The listing builds one solid part. Answer for the finished solid, in the listing's coordinates (mm). A direction names the side the tool comes from. Coordinates: 2 decimals unless noted, no trailing zeros. Loops run counter-clockwise (first coordinate to the right, second up) from the corner with the lowest first, then second, coordinate; pieces in that order, holes last. Notation, with made-up numbers: (44.25, 8) -> (77.25, 8) arc R13 cw to (77.25, 27) -> close; hole circle Ø5 at (39.25, 1). An arc over 180 degrees is marked (long way). Answer in a Markdown table with one row per item.
```python
from build123d import *

# Parameters (mm, degrees)
SKETCH1_R           = 10.5
SKETCH1_R_2         = 1.5
BOSS_EXTRUDE1_DEPTH = 2
SKETCH2_R           = 4.4
SKETCH2_R_2         = 3
BOSS_EXTRUDE2_DEPTH = 3.7
SKETCH3_R           = 0.75
CUT_EXTRUDE1_DEPTH  = 10


with BuildPart() as part:
    # Sketch1 → Boss-Extrude1 (new body)
    with BuildSketch(Plane(origin=(0, 0, 0), x_dir=(1, 0, 0), z_dir=(0, 1, 0))):
        with Locations(Location((0, 0, 0), (0, 0, 270))):
            Circle(SKETCH1_R)
        with Locations(Location((0, 0, 0), (0, 0, 270))):
            Circle(SKETCH1_R_2, mode=Mode.SUBTRACT)
    extrude(amount=-BOSS_EXTRUDE1_DEPTH)

    # Sketch2 → Boss-Extrude2 (add)
    with BuildSketch(Plane.XZ.offset(2)):
        with Locations(Location((0, 0, 0), (0, 0, 90))):
            Circle(SKETCH2_R)
        with Locations(Location((0, 0, 0), (0, 0, 270))):
            Circle(SKETCH2_R_2, mode=Mode.SUBTRACT)
    extrude(amount=BOSS_EXTRUDE2_DEPTH)

    # Sketch3 → Cut-Extrude1 (cut)
    with BuildSketch(Plane(origin=(0, 0, 0), x_dir=(1, 0, 0), z_dir=(0, 1, 0))):
        with Locations(Location((0, 7.25, 0), (0, 0, 270))):
            Circle(SKETCH3_R)
        with Locations(Location((3.5, 7.25, 0), (0, 0, 270))):
            Circle(SKETCH3_R)
        with Locations(Location((-3.5, 7.25, 0), (0, 0, 270))):
            Circle(SKETCH3_R)
        with Locations(Location((-7.25, 3.5, 0), (0, 0, 270))):
            Circle(SKETCH3_R)
        with Locations(Location((-7.25, -3.5, 0), (0, 0, 270))):
            Circle(SKETCH3_R)
        with Locations(Location((-7.25, 0, 0), (0, 0, 270))):
            Circle(SKETCH3_R)
        with Locations(Location((7.25, -3.5, 0), (0, 0, 270))):
            Circle(SKETCH3_R)
        with Locations(Location((7.25, 3.5, 0), (0, 0, 270))):
            Circle(SKETCH3_R)
        with Locations(Location((7.25, 0, 0), (0, 0, 270))):
            Circle(SKETCH3_R)
        with Locations(Location((0, -7.25, 0), (0, 0, 270))):
            Circle(SKETCH3_R)
        with Locations(Location((-3.5, -7.25, 0), (0, 0, 270))):
            Circle(SKETCH3_R)
        with Locations(Location((3.5, -7.25, 0), (0, 0, 270))):
            Circle(SKETCH3_R)
    extrude(amount=-CUT_EXTRUDE1_DEPTH, mode=Mode.SUBTRACT)


solid = part.part
```
Item 1: A tool of negligible diameter and unlimited length cuts with its end or side. For faces 4 (the face through (-1.3, -2, 1.3)), 5 (the face through (3.2, -1, 10)), from which of +Z, -Z, +X, -X, +Y, -Y can it reach the whole face along a straight path? Write none if from no direction.
Findings below:
| item | result |
|---|---|
| face 4 | -Y |
| face 5 | +Y, -Y |
Item 2: Find the intervals of material crossed by probe 1 along X at (y, z) = (-0.35, 4); probe 2 along Y at (x, z) = (-7.5, 2); probe 3 along X at (y, z) = (-1.5, 7.25), in increasing order.
Findings below:
| item | result |
|---|---|
| probe 1 | x = -9.71 to -7.81, -6.69 to 6.69, 7.81 to 9.71 |
| probe 2 | y = -2 to 0 |
| probe 3 | x = -7.6 to -4.25, -2.75 to -0.75, 0.75 to 2.75, 4.25 to 7.6 |
Item 3: A cutting plane is placed at A-A, the plane x = 0. Determine the outline of the cut face in (y, z), plus the area to 3 significant figures.
Findings below:
| item | result |
|---|---|
| outline | (-5.7, -4.4) -> (-2, -4.4) -> (-2, -6.5) -> (0, -6.5) -> (0, -1.5) -> (-2, -1.5) -> (-2, -3) -> (-5.7, -3) -> close; (-5.7, 3) -> (-2, 3) -> (-2, 1.5) -> (0, 1.5) -> (0, 6.5) -> (-2, 6.5) -> (-2, 4.4) -> (-5.7, 4.4) -> close; (-2, -10.5) -> (0, -10.5) -> (0, -8) -> (-2, -8) -> close; (-2, 8) -> (0, 8) -> (0, 10.5) -> (-2, 10.5) -> close |
| area | 40.4 mm2 |
Item 4: A cutting plane is placed at B-B, the plane z = 0. Determine the outline of the cut face in (x, y), plus the area to 3 significant figures.
Findings below:
| item | result |
|---|---|
| outline | (-10.5, -2) -> (-8, -2) -> (-8, 0) -> (-10.5, 0) -> close; (-6.5, -2) -> (-4.4, -2) -> (-4.4, -5.7) -> (-3, -5.7) -> (-3, -2) -> (-1.5, -2) -> (-1.5, 0) -> (-6.5, 0) -> close; (1.5, -2) -> (3, -2) -> (3, -5.7) -> (4.4, -5.7) -> (4.4, -2) -> (6.5, -2) -> (6.5, 0) -> (1.5, 0) -> close; (8, -2) -> (10.5, -2) -> (10.5, 0) -> (8, 0) -> close |
| area | 40.4 mm2 |
Item 5: A cutting plane is placed at D-D, the plane x = -3.25. Determine the outline of the cut face in (y, z), plus the area to 3 significant figures.
Findings below:
| item | result |
|---|---|
| outline | (-5.7, -2.97) -> (-2, -2.97) -> (-2, -6.54) -> (0, -6.54) -> (0, 6.54) -> (-2, 6.54) -> (-2, 2.97) -> (-5.7, 2.97) -> close; (-2, -9.98) -> (0, -9.98) -> (0, -7.96) -> (-2, -7.96) -> close; (-2, 7.96) -> (0, 7.96) -> (0, 9.98) -> (-2, 9.98) -> close |
| area | 56.2 mm2 |
Item 6: Determine the mould class of faces 1 (the face through (0, 0, 2)), 2 (the face through (-4.363, -3.824, -0.573)), 3 (the face through (0.9, -3.82, -2.86)) for opening direction X: +X half, -X half, draft (parallel to the pull), parting line (faces both ways), or undercut.
Findings below:
| item | result |
|---|---|
| face 1 | draft |
| face 2 | parting line |
| face 3 | undercut |
Item 7: Flat-ended cylindrical pins translate along their axes: pin 1 Ø3 at (y, z) = (-1.5, -8.5) entering from -X; pin 2 Ø1.2 at (x, z) = (7.25, 0) entering from +Y; pin 3 Ø3.5 at (x, z) = (0, 0) entering from -Y; pin 4 Ø1.5 at (y, z) = (-2.5, -3) entering from -X. Find the tip coordinate at first contact, or state that the pin passes through.
Findings below:
| item | result |
|---|---|
| pin 1 | stops at x = -7.83 |
| pin 2 | passes through |
| pin 3 | stops at y = -2 |
| pin 4 | stops at x = -10.21 |
Item 8: A cutting plane is placed at C-C, the plane z = -3.25. Determine the outline of the cut face in (x, y), plus the area to 3 significant figures.
Findings below:
| item | result |
|---|---|
| outline | (-9.98, -2) -> (-7.96, -2) -> (-7.96, 0) -> (-9.98, 0) -> close; (-6.54, -2) -> (-2.97, -2) -> (-2.97, -5.7) -> (2.97, -5.7) -> (2.97, -2) -> (6.54, -2) -> (6.54, 0) -> (-6.54, 0) -> close; (7.96, -2) -> (9.98, -2) -> (9.98, 0) -> (7.96, 0) -> close |
| area | 56.2 mm2 |
